Can you work these out from the model? Positions are in its coordinate system, mm. A direction names the side the tool comes from. Coordinates: 2 decimals unless noted, no trailing zeros. Write each loop counter-clockwise with the first axis right and the second up, starting at its lowest first coordinate (ties: lowest second). Pieces come first, ordered by that corner, then holes. Notation, with made-up numbers: (-30.75, -1) -> (7.25, -1) arc R13 cw to (7.25, 16) -> close; hole circle Ø7 at (49.5, 86). An arc over 180 degrees is marked (long way). Use one line per item in the form item = value.
```python
from build123d import *

# Parameters (mm, degrees)
F0_W     = 177.8
F0_H     = 12.7
F1_DEPTH = 12.7
F2_R     = 1.27
F3_W     = 5.08
F3_H     = 7.62
F4_DEPTH = 177.8
F5_R     = 1.26999


# Not quite as in the source:
# - a fillet or chamfer is up to 0.001 mm smaller than in the source, because OpenCascade refuses the exact size


with BuildPart() as f1:
    # F0 (on Top) → F1 (new body)
    with BuildSketch(Plane.XY):
        Rectangle(F0_W, F0_H)
    extrude(amount=F1_DEPTH)

    # F2
    f2_edges = [f1.edges().sort_by_distance(p)[0] for p in [
        (0, 6.35, 0),
        (0, -6.35, 12.7),
        (0, -6.35, 0),
        (0, 6.35, 12.7),
    ]]
    fillet(f2_edges, radius=F2_R)

    # F3 (on face) → F4 (cut)
    with BuildSketch(Plane.YZ.offset(88.9)):
        with Locations((-3.81, 6.35)):
            Rectangle(F3_W, F3_H)
        with Locations((3.81, 6.35)):
            Rectangle(F3_W, F3_H)
    extrude(amount=-F4_DEPTH, mode=Mode.SUBTRACT)

    # F5 (radius 1.27 in the source; OpenCascade refuses exactly that, so slightly less here)
    f5_edges = [f1.edges().sort_by_distance(p)[0] for p in [
        (0, -6.35, 10.16),
        (0, -6.35, 2.54),
        (0, 6.35, 10.16),
        (0, 6.35, 2.54),
    ]]
    fillet(f5_edges, radius=F5_R)


solid = f1.part
```
Q1. For faces 4 (the flat face through (1, -3, 10.16)), 5 (the flat face through (1, 3, 2.54)), 6 (the flat face through (-88.9, 0, 6)), which set-ups out of +Z, -Z, +X, -X, +Y, -Y let a thin tool reach every point of the face, with its end or its side?
Return value:
face_4 = +X, -X, -Y
face_5 = +X, -X, +Y
face_6 = +Z, -Z, -X, +Y, -Y
Q2. Will this pin go through, and if not, where does the flat tip stop? pin 1 (1 mm diameter, centred on x = -66, z = 2.5, fed in from -Y).
Return value:
pin_1 = -6.12
Q3. Suppose I cut it at A-A (y = -3). Write out the boundary of the cut face in (x, z).
Return value:
outline = (-88.9, 0) -> (88.9, 0) -> (88.9, 2.54) -> (-88.9, 2.54) -> close; (-88.9, 10.16) -> (88.9, 10.16) -> (88.9, 12.7) -> (-88.9, 12.7) -> close
Q4. If I drill on line 1 (Z direction, x = -12.5, y = -2); line 2 (Y direction, x = 44, z = 5.5); line 3 (Y direction, x = 50, z = 11.5), over which ranges is the centre line in solid material (lowest first)? Write a range as from..to.
Return value:
line_1 = 0..2.54, 10.16..12.7
line_2 = -1.27..1.27
line_3 = -6.35..6.35
Q5. Thinking about a two-plate mould opening in Z: for faces 1 (the flat face through (-1, 0, 0)), 2 (the flat face through (1, -3, 2.54)), 3 (the flat face through (-1, 0, 12.7)), which applies, released by +Z, released by -Z, zero draft, split by the parting line, or undercut?
Return value:
face_1 = released by -Z
face_2 = undercut
face_3 = released by +Z
Q6. Suppose I cut it at C-C (z = 4.75). Write out the boundary of the cut face in (x, y).
Return value:
outline = (-88.9, -1.27) -> (88.9, -1.27) -> (88.9, 1.27) -> (-88.9, 1.27) -> close
